from build123d import *

# Parameters (mm, degrees)
F0_W     = 110
F0_H     = 70
F1_DEPTH = 25
F2_W     = 107.6
F2_H     = 67.6
F3_DEPTH = 23.8
F4_R     = 3


with BuildPart() as f1:
    # F0 (on Top) → F1 (new body)
    with BuildSketch(Plane.XY):
        Rectangle(F0_W, F0_H)
    extrude(amount=F1_DEPTH)

    # F2 (on face) → F3 (cut)
    with BuildSketch(Plane.XY.offset(25)):
        Rectangle(F2_W, F2_H)
    extrude(amount=-F3_DEPTH, mode=Mode.SUBTRACT)

    # F4
    f4_edges = [f1.edges().sort_by_distance(p)[0] for p in [
        (-53.8, 33.8, 13.1),
        (-53.8, 0, 1.2),
        (0, 33.8, 1.2),
        (53.8, 33.8, 13.1),
        (53.8, 0, 1.2),
        (53.8, -33.8, 13.1),
        (0, -33.8, 1.2),
        (-53.8, -33.8, 13.1),
    ]]
    fillet(f4_edges, radius=F4_R)


solid = f1.part
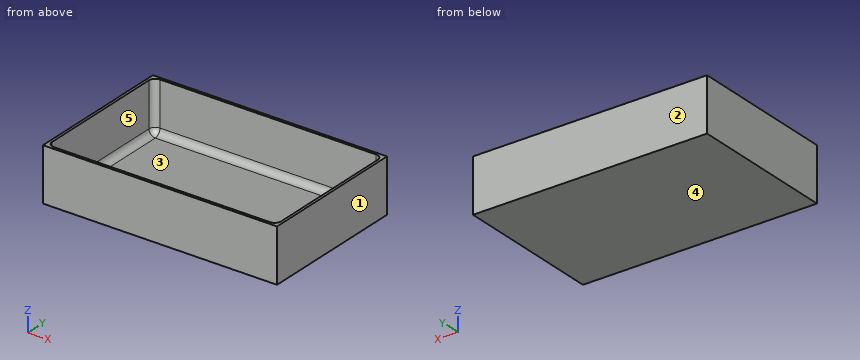
Model file for the job. Use its own axes, mm. Face numbers are marked on the shaded views. A direction names the side the tool comes from. Give positions to 0.01 mm unless a question says otherwise; leave off trailing zeros. Order: outer loops, then holes, each group sorted by start corner. A loop starts at its lowest first (then second) coordinate and runs counter-clockwise, first axis right, second up. Notation, with made-up numbers: (83.25, 86) - (112.25, 86) arc R26 ccw to (112.25, 107) - close; hole circle Ø3 at (25.5, 38.5). An arc over 180 degrees is marked (long way). Write item = value, one per line. Start each with the question number.
1. Probe line 1 along Y through (x, z) = (-40, 13); line 2 along X through (y, z) = (-31, 20.75); line 3 along Z through (x, y) = (33.5, 30.5). List the from-to ranges inside material, lowest first.
2. Drop a flat-ended pin along its axis: P1, Ø5, axis at x = 1, y = 11, coming from the +Z side. Give the stop position or say it passes through.
3. Two-plate mould, pull along X, no slides. Class the marked faces 1, 2 and 3: pulls with the +X half, pulls with the -X half, needs draft (parallel to the pull), parting line crosses it, or undercut.
4. Which spindle directions (+Z, -Z, +X, -X, +Y, -Y) get a long thin tool onto all of the face, cutting with end or side? Do the marked faces 4 and 5. Say none if no direction does.
5. Cut at D-D, the plane z = 2.5. List the corners of the cut face in (x, y).
6. Cut at A-A, the plane z = 21.25. List the corners of the cut face in (x, y).
7. Cut at B-B, the plane y = 3.5. List the corners of the cut face in (x, z).
8. Cut at C-C, the plane x = 48. List the corners of the cut face in (y, z).
Taken from the geometry:
q1.line_1 = -35 to -33.8, 33.8 to 35
q1.line_2 = -55 to -53.79, 53.79 to 55
q1.line_3 = 0 to 1.2
q2.P1 = 1.2
q3.face_1 = pulls with the +X half
q3.face_2 = needs draft
q3.face_3 = undercut
q4.face_4 = -Z, +X, -X, +Y, -Y
q4.face_5 = +Z
q5.outline = (-55, -35) - (55, -35) - (55, 35) - (-55, 35) - close; hole (-53.27, -30.8) arc R2.47 ccw to (-50.8, -33.27) - (50.8, -33.27) arc R2.47 ccw to (53.27, -30.8) - (53.27, 30.8) arc R2.47 ccw to (50.8, 33.27) - (-50.8, 33.27) arc R2.47 ccw to (-53.27, 30.8) - close
q6.outline = (-55, -35) - (55, -35) - (55, 35) - (-55, 35) - close; hole (-53.8, -30.8) arc R3 ccw to (-50.8, -33.8) - (50.8, -33.8) arc R3 ccw to (53.8, -30.8) - (53.8, 30.8) arc R3 ccw to (50.8, 33.8) - (-50.8, 33.8) arc R3 ccw to (-53.8, 30.8) - close
q7.outline = (-55, 0) - (55, 0) - (55, 25) - (53.8, 25) - (53.8, 4.2) arc R3 cw to (50.8, 1.2) - (-50.8, 1.2) arc R3 cw to (-53.8, 4.2) - (-53.8, 25) - (-55, 25) - close
q8.outline = (-35, 0) - (35, 0) - (35, 25) - (33.8, 25) - (33.8, 4.2) arc R3 cw to (30.8, 1.2) - (-30.8, 1.2) arc R3 cw to (-33.8, 4.2) - (-33.8, 25) - (-35, 25) - close
